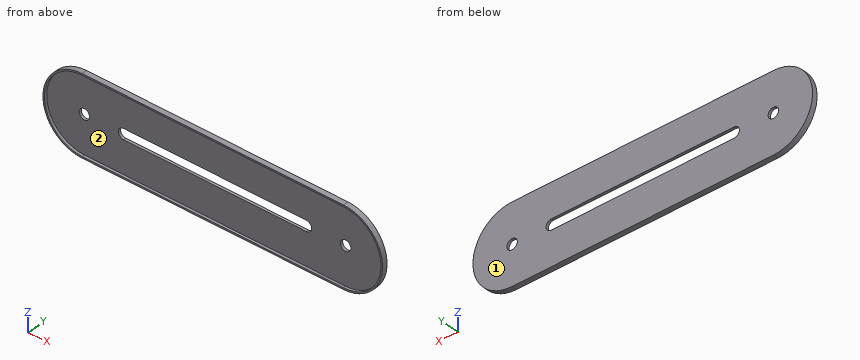
from build123d import *

# Parameters (mm, degrees)
SKETCH1_R           = 10
BOSS_EXTRUDE1_DEPTH = 5
CUT_EXTRUDE1_DEPTH  = 5


with BuildPart() as part:
    # Sketch1 → Boss-Extrude1 (new, symmetric)
    with BuildSketch(Plane(origin=(0, 0, 0), x_dir=(-1, 0, 0), z_dir=(0, 1, 0))):
        with BuildLine():
            Line((-250, 75), (250, 75))
            ThreePointArc((250, 75), (325, 0), (250, -75))
            Line((250, -75), (-250, -75))
            ThreePointArc((-250, -75), (-325, 0), (-250, 75))
        make_face()
        with Locations(Location((250, 0, 0), (0, 0, 90))):
            Circle(SKETCH1_R, mode=Mode.SUBTRACT)
        with Locations(Location((-250, 0, 0), (0, 0, 270))):
            Circle(SKETCH1_R, mode=Mode.SUBTRACT)
        with BuildLine():
            Line((-175, 10), (175, 10))
            ThreePointArc((175, 10), (185, 0), (175, -10))
            Line((175, -10), (-175, -10))
            ThreePointArc((-175, -10), (-185, 0), (-175, 10))
        make_face(mode=Mode.SUBTRACT)
    extrude(amount=BOSS_EXTRUDE1_DEPTH, both=True)

    # Sketch4 → Cut-Extrude1 (cut)
    with BuildSketch(Plane.XZ.offset(5)):
        with BuildLine():
            Line((250, 72), (-250, 72))
            ThreePointArc((-250, 72), (-322, 0), (-250, -72))
            Line((-250, -72), (250, -72))
            ThreePointArc((250, -72), (322, 0), (250, 72))
        make_face()
    extrude(amount=-CUT_EXTRUDE1_DEPTH, mode=Mode.SUBTRACT)


solid = part.part
Build history of the part. All positions in model axes, mm. Face numbers are marked on the shaded views. A direction names the side the tool comes from. Round coordinates to 2 decimals unless told otherwise and drop trailing zeros. Write each loop counter-clockwise with the first axis right and the second up, starting at its lowest first coordinate (ties: lowest second). Pieces come first, ordered by that corner, then holes. Notation, with made-up numbers: M 80,-36.75 L 127,-36.75 A16 cw 127,-6.75 Z; hole C -37,74.25 d6. An arc over 180 degrees is marked long. Answer as a JSON object with one key per item and string values. Group by question number.
(1) Cut at B-B (z = 0). Give the cut face in (x, y).
(2) Which spindle directions (+Z, -Z, +X, -X, +Y, -Y) get a long thin tool onto all of the face, cutting with end or side? Do the marked faces 1 and 2. Say none if no direction does.
(3) Flat gauge pins, fed straight in: pin 1 (6 mm diameter, centred on y = -3, z = -30, fed in from +X); pin 2 (2 mm diameter, centred on y = -3, z = -9.5, fed in from -X); pin 3 (1 mm diameter, centred on y = 3, z = 46, fed in from -X). Where does each tip first touch, or does it go through?
(4) Cut at A-A (x = 118). Give the cut face in (y, z).
(5) Cut at D-D (x = -191). Give the cut face in (y, z), and give its area (3 significant figures).
(6) Drill centre lines: L1, parallel to X at y = 3.8, z = 0; L2, parallel to Z at x = 54, y = -2.5; L3, parallel to Z at x = -97, y = 4. Where is each one in solid material? Low to high.
(7) Cut at C-C (y = -2.75). Give the cut face in (x, z), and give its area (3 significant figures).
Responses:
{
 "1": {"outline": "M -325,-5 L -322,-5 L -322,0 L -260,0 L -260,5 L -325,5 Z; M -240,0 L -185,0 L -185,5 L -240,5 Z; M 185,0 L 240,0 L 240,5 L 185,5 Z; M 260,0 L 322,0 L 322,-5 L 325,-5 L 325,5 L 260,5 Z"},
 "2": {"face 1": "+Z, -Z, +X, -X, +Y", "face 2": "-Y"},
 "3": {"pin 1": "stops at x = 319.97", "pin 2": "stops at x = -324.52", "pin 3": "stops at x = -309.62"},
 "4": {"outline": "M -5,-75 L 5,-75 L 5,-10 L 0,-10 L 0,-72 L -5,-72 Z; M -5,72 L 0,72 L 0,10 L 5,10 L 5,75 L -5,75 Z"},
 "5": {"outline": "M -5,-75 L 5,-75 L 5,75 L -5,75 L -5,72 L 0,72 L 0,-72 L -5,-72 Z", "area": "780 mm2"},
 "6": {"L1": "x = -325 to -260, -240 to -185, 185 to 240, 260 to 325", "L2": "z = -75 to -72, 72 to 75", "L3": "z = -75 to -10, 10 to 75"},
 "7": {"outline": "M -250,-75 L 250,-75 A75 ccw 250,75 L -250,75 A75 ccw Z; hole M -250,-72 L 250,-72 A72 ccw 250,72 L -250,72 A72 ccw Z", "area": "4,390 mm2"}
}
